Input: part model. Units: mm. Frame: model coordinates. Face numbers are marked on the shaded views. A direction names the side the tool comes from. Coordinates: 2 decimals unless noted, no trailing zeros. Order: outer loops, then holes, each group sorted by start corner. A loop starts at its lowest first (then second) coordinate and runs counter-clockwise, first axis right, second up. Notation, with made-up numbers: M -12,7 L -8,7 A23 ccw -8,38 Z; hole C -10,20.25 d8. An arc over 180 degrees is marked long. One line per item, written item: value.
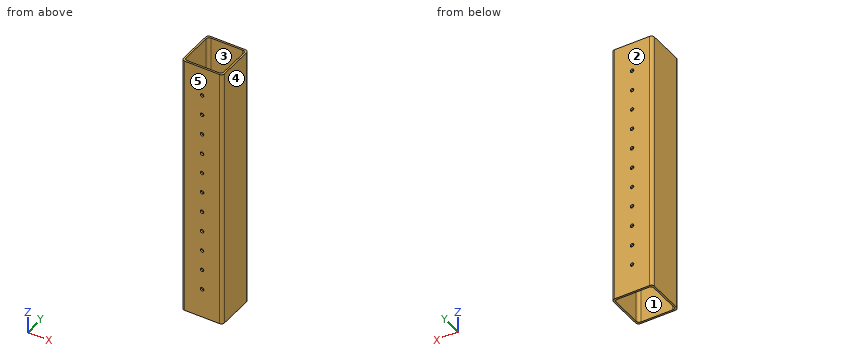
```python
from build123d import *

# Parameters (mm, degrees)
SKETCH1_W           = 70
SKETCH1_H           = 70
SKETCH1_W_2         = 64
SKETCH1_H_2         = 64
BOSS_EXTRUDE1_DEPTH = 450
FILLET1_R           = 5
SKETCH3_R           = 3
CUT_EXTRUDE2_DEPTH  = 173
LPATTERN1_COUNT     = 6
LPATTERN1_PITCH     = 35
LPATTERN1_COL_COUNT = 6
LPATTERN1_COL_PITCH = 35


with BuildPart() as part:
    # Sketch1 → Boss-Extrude1 (new body)
    with BuildSketch(Plane.XY):
        with Locations((35, 35)):
            Rectangle(SKETCH1_W, SKETCH1_H)
        with Locations((35, 35)):
            Rectangle(SKETCH1_W_2, SKETCH1_H_2, mode=Mode.SUBTRACT)
    extrude(amount=BOSS_EXTRUDE1_DEPTH)

    # Fillet1
    fillet1_edges = [part.edges().sort_by_distance(p)[0] for p in [
        (3, 67, 225),
        (3, 3, 225),
        (67, 3, 225),
        (67, 67, 225),
        (0, 70, 225),
        (70, 70, 225),
        (70, 0, 225),
        (0, 0, 225),
    ]]
    fillet(fillet1_edges, radius=FILLET1_R)

    # Sketch3 → Cut-Extrude2 (cut)
    with BuildSketch(Plane.XZ):
        with Locations(Location((35, 225, 0), (0, 0, 270))):
            Circle(SKETCH3_R)
    cut_extrude2 = extrude(amount=-CUT_EXTRUDE2_DEPTH, mode=Mode.SUBTRACT)

    # LPattern1: Cut-Extrude2 ×6
    with Locations(*[(0, 0, -i * LPATTERN1_PITCH) for i in range(1, LPATTERN1_COUNT)]):
        add(cut_extrude2, mode=Mode.SUBTRACT)

    # LPattern1 col: Cut-Extrude2 ×6
    with Locations(*[(0, 0, i * LPATTERN1_COL_PITCH) for i in range(1, LPATTERN1_COL_COUNT)]):
        add(cut_extrude2, mode=Mode.SUBTRACT)


solid = part.part
```
(1) Cut plane A-A on x = 50.5. Output: boundary loops of the cut face in (y, z).
Data:
outline: M 0,0 L 3,0 L 3,450 L 0,450 Z; M 67,0 L 70,0 L 70,450 L 67,450 Z
(2) Cut plane C-C on z = 349. Output: boundary loops of the cut face in (x, y), plus the area to 3 significant figures.
Data:
outline: M 0,5 A5 ccw 5,0 L 65,0 A5 ccw 70,5 L 70,65 A5 ccw 65,70 L 5,70 A5 ccw 0,65 Z; hole M 3,8 A5 ccw 8,3 L 62,3 A5 ccw 67,8 L 67,62 A5 ccw 62,67 L 8,67 A5 ccw 3,62 Z
area: 804 mm2
(3) First-contact query: pin 1 (7 mm diameter, centred on x = 35, z = 225, fed in from +Y). Flat tip, straight axial feed; report the tip coordinate or a pass-through.
Data:
pin 1: stops at y = 70
(4) Draft query along Y for the marked faces 3, 4 and 5. Return one class per face: released by +Y, released by -Y, zero draft, split by the parting line, or undercut.
Data:
face 3: undercut
face 4: zero draft
face 5: released by -Y
(5) Ray query, line 1 (X direction, y = 50, z = 65.5); line 2 (Y direction, x = 66, z = 230). Return the intervals inside material, ascending. Write a range as from..to.
Data:
line 1: x = 0..3, 67..70
line 2: y = 0.1..5, 65..69.9
(6) Access query for the marked faces 1 and 2. Directions: +Z, -Z, +X, -X, +Y, -Y. A direction counts if a zero-diameter tool reaches every point of the face in a straight line with its end or side. Return the directions, or none.
Data:
face 1: +Z, -Z
face 2: +Z, -Z, +X, -X, +Y
